Design review of the part built by this model. Coordinates are the model's own, in mm. A direction names the side the tool comes from. Give positions to 0.01 mm unless a question says otherwise; leave off trailing zeros. Loops run counter-clockwise (first coordinate to the right, second up) from the corner with the lowest first, then second, coordinate; pieces in that order, holes last. Notation, with made-up numbers: (36, 34) -> (85, 34) arc R31 cw to (85, 62) -> close; hole circle Ø7 at (-9.5, -5.5). An arc over 180 degrees is marked (long way). Use a Markdown table: item, result. Add a question column.
1. To check wall thickness, follow line 1 (X direction, y = -0.5, z = 3.5); line 2 (X direction, y = -1, z = 1); line 3 (Z direction, x = -13, y = -5.25). State the ranges of each line that lie inside material, in increasing order.
2. For pin 1 Ø0.8 at (x, y) = (18, -0.5) entering from +Z; pin 2 Ø12 at (x, y) = (-11, 0) entering from +Z; pin 3 Ø10 at (x, y) = (4.5, -4.5) entering from +Z, all flat-tipped, find the tip position at first contact; note any pin that passes through.
3. Draft analysis for pull direction Y (two halves, no side actions). For faces 1 (the flat face through (0, -15, 6.3)), 2 (the cylindrical face through (-21.7, 6.7, 3.5)), 3 (the flat face through (-17, 5, 2)), state which applies: pulls with the +Y half, pulls with the -Y half, needs draft (parallel to the pull), parting line crosses it, or undercut.
4. Add section B-B (y = 2.5). State the section outline as (x, z) points, and give its area (3 significant figures).
5. Add section C-C (x = 15). State the section outline as (y, z) points.
6. Add section A-A (x = 2.5). State the section outline as (y, z) points.
7. For faces 4 (the flat face through (19.5, 0, 0)), 5 (the flat face through (-19.5, 0, 0)), 6 (the flat face through (17, 0, 1.5)), 7 (the flat face through (13, -9, 2)), list the 3-axis set-ups (+Z, -Z, +X, -X, +Y, -Y) from which the entire face can be reached by the end or side of a thin tool; tool diameter is ignored.
8. Add section D-D (y = -7.25). State the section outline as (x, z) points.
```python
from build123d import *

# Parameters (mm, degrees)
SKETCH1_W           = 1
SKETCH1_H           = 2.5
SKETCH1_W_2         = 10
SKETCH1_H_2         = 3.5
BOSS_EXTRUDE1_DEPTH = 1
BOSS_EXTRUDE2_START = 4.3
SKETCH1_3_W         = 1
SKETCH1_3_H         = 2.5
BOSS_EXTRUDE2_DEPTH = 4.3
CUT_EXTRUDE1_REACH  = 29.14
CUT_EXTRUDE2_DEPTH  = 33.393667716
BOSS_EXTRUDE4_START = 2
BOSS_EXTRUDE4_DEPTH = 2
SKETCH3_5_W         = 1
SKETCH3_5_H         = 0.8
BOSS_EXTRUDE5_DEPTH = 2.5


with BuildPart() as part:
    # Sketch1 → Boss-Extrude1 (new body)
    # profile 1 of 4: a face of its own
    with BuildSketch(Plane(origin=(0, 0, 0), x_dir=(-1, 0, 0), z_dir=(0, 0, 1))):
        with BuildLine():
            ThreePointArc((-20.5, -7.1), (-21.914213562, -6.514213562), (-22.5, -5.1))
            Line((-22.5, -5.1), (-22.5, 4.115748324))
            ThreePointArc((-22.5, 4.115748324), (0, 15.804360023), (22.5, 4.115748324))
            Line((22.5, 4.115748324), (22.5, -5.1))
            ThreePointArc((22.5, -5.1), (21.914213562, -6.514213562), (20.5, -7.1))
            Line((20.5, -7.1), (-20.5, -7.1))
        make_face()
        with BuildLine():
            Line((-13, 6.3), (-13, 10.821020521))
            ThreePointArc((-13, 10.821020521), (0, 14.304360023), (13, 10.821020521))
            Line((13, 10.821020521), (13, 6.3))
            Line((13, 6.3), (17, 6.3))
            Line((17, 6.3), (17, 3))
            Line((17, 3), (19.3, 3))
            Line((19.3, 3), (19.3, -3))
            Line((19.3, -3), (17, -3))
            Line((17, -3), (17, -6.1))
            Line((17, -6.1), (-17, -6.1))
            Line((-17, -6.1), (-17, -3))
            Line((-17, -3), (-19.3, -3))
            Line((-19.3, -3), (-19.3, 3))
            Line((-19.3, 3), (-17, 3))
            Line((-17, 3), (-17, 6.3))
            Line((-17, 6.3), (-13, 6.3))
        make_face(mode=Mode.SUBTRACT)
    # profile 2 of 4: a face of its own
    with BuildSketch(Plane(origin=(0, 0, 0), x_dir=(-1, 0, 0), z_dir=(0, 0, 1))):
        with BuildLine():
            ThreePointArc((-13, 10.821020521), (0, 14.304360023), (13, 10.821020521))
            Line((13, 10.821020521), (13, 6.3))
            Line((13, 6.3), (17, 6.3))
            Line((17, 6.3), (17, 3))
            Line((17, 3), (19.3, 3))
            Line((19.3, 3), (19.3, -3))
            Line((19.3, -3), (17, -3))
            Line((17, -3), (17, -6.1))
            Line((17, -6.1), (-17, -6.1))
            Line((-17, -6.1), (-17, -3))
            Line((-17, -3), (-19.3, -3))
            Line((-19.3, -3), (-19.3, 3))
            Line((-19.3, 3), (-17, 3))
            Line((-17, 3), (-17, 6.3))
            Line((-17, 6.3), (-13, 6.3))
            Line((-13, 6.3), (-13, 10.821020521))
        make_face()
        with Locations((-18, 0)):
            Rectangle(SKETCH1_W, SKETCH1_H, mode=Mode.SUBTRACT)
        with Locations((0, 3.65)):
            Rectangle(SKETCH1_W_2, SKETCH1_H_2, mode=Mode.SUBTRACT)
        with Locations((18, 0)):
            Rectangle(SKETCH1_W, SKETCH1_H, mode=Mode.SUBTRACT)
    # profile 3 of 4: a face of its own
    with BuildSketch(Plane(origin=(0, 0, 0), x_dir=(-1, 0, 0), z_dir=(0, 0, 1))):
        with Locations((18, 0)):
            Rectangle(SKETCH1_W, SKETCH1_H)
    # profile 4 of 4: a face of its own
    with BuildSketch(Plane(origin=(0, 0, 0), x_dir=(-1, 0, 0), z_dir=(0, 0, 1))):
        with Locations((-18, 0)):
            Rectangle(SKETCH1_W, SKETCH1_H)
    extrude(amount=-BOSS_EXTRUDE1_DEPTH)

    # Sketch1<3> → Boss-Extrude2 (add)
    # profile 1 of 3: a face of its own
    with BuildSketch(Plane(origin=(0, 0, 0), x_dir=(-1, 0, 0), z_dir=(0, 0, 1)).offset(BOSS_EXTRUDE2_START)):
        with BuildLine():
            ThreePointArc((-20.5, -7.1), (-21.914213562, -6.514213562), (-22.5, -5.1))
            Line((-22.5, -5.1), (-22.5, 4.115748324))
            ThreePointArc((-22.5, 4.115748324), (0, 15.804360023), (22.5, 4.115748324))
            Line((22.5, 4.115748324), (22.5, -5.1))
            ThreePointArc((22.5, -5.1), (21.914213562, -6.514213562), (20.5, -7.1))
            Line((20.5, -7.1), (-20.5, -7.1))
        make_face()
        with BuildLine():
            Line((-13, 6.3), (-13, 10.821020521))
            ThreePointArc((-13, 10.821020521), (0, 14.304360023), (13, 10.821020521))
            Line((13, 10.821020521), (13, 6.3))
            Line((13, 6.3), (17, 6.3))
            Line((17, 6.3), (17, 3))
            Line((17, 3), (19.3, 3))
            Line((19.3, 3), (19.3, -3))
            Line((19.3, -3), (17, -3))
            Line((17, -3), (17, -6.1))
            Line((17, -6.1), (-17, -6.1))
            Line((-17, -6.1), (-17, -3))
            Line((-17, -3), (-19.3, -3))
            Line((-19.3, -3), (-19.3, 3))
            Line((-19.3, 3), (-17, 3))
            Line((-17, 3), (-17, 6.3))
            Line((-17, 6.3), (-13, 6.3))
        make_face(mode=Mode.SUBTRACT)
    # profile 2 of 3: a face of its own
    with BuildSketch(Plane(origin=(0, 0, 0), x_dir=(-1, 0, 0), z_dir=(0, 0, 1)).offset(BOSS_EXTRUDE2_START)):
        with Locations((18, 0)):
            Rectangle(SKETCH1_3_W, SKETCH1_3_H)
    # profile 3 of 3: a face of its own
    with BuildSketch(Plane(origin=(0, 0, 0), x_dir=(-1, 0, 0), z_dir=(0, 0, 1)).offset(BOSS_EXTRUDE2_START)):
        with Locations((-18, 0)):
            Rectangle(SKETCH1_3_W, SKETCH1_3_H)
    extrude(amount=-BOSS_EXTRUDE2_DEPTH)

    # Sketch3 → Cut-Extrude1 (cut, up to next)
    with BuildSketch(Plane.XZ.offset(1.25), mode=Mode.PRIVATE) as cut_extrude1_sk1:
        with BuildLine():
            Line((-17.5, 0), (-17.5, 1))
            ThreePointArc((-17.5, 1), (-17.633974596, 0.5), (-17.5, 0))
        make_face()
    cut_extrude1_tool1 = extrude(cut_extrude1_sk1.sketch, amount=-CUT_EXTRUDE1_REACH, mode=Mode.PRIVATE) & part.part
    # Sketch3 → Cut-Extrude1 (cut, up to next)
    with BuildSketch(Plane.XZ.offset(1.25), mode=Mode.PRIVATE) as cut_extrude1_sk2:
        with BuildLine():
            ThreePointArc((17.5, 0), (17.633974596, 0.5), (17.5, 1))
            Line((17.5, 1), (17.5, 0))
        make_face()
    cut_extrude1_tool2 = extrude(cut_extrude1_sk2.sketch, amount=-CUT_EXTRUDE1_REACH, mode=Mode.PRIVATE) & part.part
    add(cut_extrude1_tool1.solids().sort_by_distance((-17.55391, -1.25, 0.5))[0], mode=Mode.SUBTRACT)
    add(cut_extrude1_tool2.solids().sort_by_distance((17.55391, -1.25, 0.5))[0], mode=Mode.SUBTRACT)

    # Sketch4 → Cut-Extrude2 (cut, through all)
    with BuildSketch(Plane(origin=(0, 7.1, 0), x_dir=(1, 0, 0), z_dir=(0, 1, 0))):
        Polygon((19.5, 1), (19.5, -0.3), (22.5, -3.3), (22.5, 1), align=None)
        Polygon((-19.5, -0.3), (-22.5, -3.3), (-22.5, 1), (-19.5, 1), align=None)
    extrude(amount=-CUT_EXTRUDE2_DEPTH, mode=Mode.SUBTRACT)

    # Sketch5 → Boss-Extrude4 (add)
    with BuildSketch(Plane.XY.offset(4.3).offset(BOSS_EXTRUDE4_START)):
        with BuildLine():
            Line((17, -7.976675596), (17, -9.920326344))
            ThreePointArc((17, -9.920326344), (0, -15.804360023), (-17, -9.920326344))
            Line((-17, -9.920326344), (-17, -7.976675596))
            ThreePointArc((-17, -7.976675596), (0, -14.304360023), (17, -7.976675596))
        make_face()
    extrude(amount=-BOSS_EXTRUDE4_DEPTH)

    # Sketch3<5> → Boss-Extrude5 (add)
    with BuildSketch(Plane.XZ.offset(1.25)):
        with Locations((17, 2.4)):
            Rectangle(SKETCH3_5_W, SKETCH3_5_H)
        Polygon((16.5, 2), (17.5, 2), (17.5, 1), align=None)
        with Locations((-17, 2.4)):
            Rectangle(SKETCH3_5_W, SKETCH3_5_H)
        Polygon((-16.5, 2), (-17.5, 2), (-17.5, 1), align=None)
    extrude(amount=-BOSS_EXTRUDE5_DEPTH)


solid = part.part
```
Taken from the geometry:
| question | item | result |
|---|---|---|
| 1 | line 1 | x = -22.5 to -19.3, -18.5 to -17.5, 17.5 to 18.5, 19.3 to 22.5 |
| 1 | line 2 | x = -20.2 to -19.3, -18.5 to -17.5, 17.5 to 18.5, 19.3 to 20.2 |
| 1 | line 3 | z = -1 to 0 |
| 2 | pin 1 | stops at z = 4.3 |
| 2 | pin 2 | stops at z = 2.8 |
| 2 | pin 3 | stops at z = 0 |
| 3 | face 1 | needs draft |
| 3 | face 2 | pulls with the +Y half |
| 3 | face 3 | undercut |
| 4 | outline | (-22.5, 3.3) -> (-19.5, 0.3) -> (-19.5, -1) -> (19.5, -1) -> (19.5, 0.3) -> (22.5, 3.3) -> (22.5, 4.3) -> (19.3, 4.3) -> (19.3, 0) -> (-19.3, 0) -> (-19.3, 4.3) -> (-22.5, 4.3) -> close |
| 4 | area | 55.7 mm^2 |
| 5 | outline | (-11.35, -1) -> (7.1, -1) -> (7.1, 4.3) -> (6.1, 4.3) -> (6.1, 0) -> (-6.3, 0) -> (-6.3, 4.3) -> (-9.54, 4.3) -> (-9.54, 6.3) -> (-11.35, 6.3) -> close |
| 6 | outline | (-15.69, -1) -> (-5.4, -1) -> (-5.4, 0) -> (-14.18, 0) -> (-14.18, 6.3) -> (-15.69, 6.3) -> close; (-1.9, -1) -> (7.1, -1) -> (7.1, 4.3) -> (6.1, 4.3) -> (6.1, 0) -> (-1.9, 0) -> close |
| 7 | face 4 | -Z, +X, +Y, -Y |
| 7 | face 5 | -Z, -X, +Y, -Y |
| 7 | face 6 | none |
| 7 | face 7 | +Z |
| 8 | outline | (-19.93, 0.73) -> (-19.5, 0.3) -> (-19.5, -1) -> (19.5, -1) -> (19.5, 0.3) -> (19.93, 0.73) -> (19.93, 4.3) -> (13, 4.3) -> (13, 0) -> (-13, 0) -> (-13, 4.3) -> (-19.93, 4.3) -> close |
